```python
from build123d import *

# Parameters (mm, degrees)
CONG_1_R = 0.3


with BuildPart() as part:
    # Esquisse1 → Base-Révolution (revolve)
    with BuildSketch(Plane.XY):
        with BuildLine():
            Line((3.618033989, 3.25), (5, 3.25))
            Line((5, 3.25), (5, 2))
            Line((5, 2), (0, 2))
            Line((0, 2), (0, 3.25))
            Line((0, 3.25), (1.381966011, 3.25))
            ThreePointArc((1.381966011, 3.25), (2.5, 2.75), (3.618033989, 3.25))
        make_face()
    revolve(axis=Axis((0, 0, 0), (1, 0, 0)))

    # Congé1
    cong_1_edges = [part.edges().sort_by_distance(p)[0] for p in [
        (5, -2, 0),
        (0, -2, 0),
    ]]
    fillet(cong_1_edges, radius=CONG_1_R)


solid = part.part
```
Could you check a few things on this model? Use its own coordinates, in mm. Coordinates: 2 decimals unless noted, no trailing zeros. Write each loop counter-clockwise with the first axis right and the second up, starting at its lowest first coordinate (ties: lowest second). Pieces come first, ordered by that corner, then holes. Notation, with made-up numbers: (79.25, 28) - (96.25, 28) arc R25 ccw to (96.25, 42) - close; hole circle Ø2 at (44.5, 81). An arc over 180 degrees is marked (long way). Use a Markdown table: item, result.
Q1. Imagine slicing it at A-A (z = 0). List the corners of the cut face in (x, y) for me, and give its area (3 significant figures).
Geometry check:
| item | result |
|---|---|
| outline | (0, -3.25) - (1.38, -3.25) arc R1.5 cw to (3.62, -3.25) - (5, -3.25) - (5, -2.3) arc R0.3 ccw to (4.7, -2) - (0.3, -2) arc R0.3 ccw to (0, -2.3) - close; (0, 2.3) arc R0.3 ccw to (0.3, 2) - (4.7, 2) arc R0.3 ccw to (5, 2.3) - (5, 3.25) - (3.62, 3.25) arc R1.5 cw to (1.38, 3.25) - (0, 3.25) - close |
| area | 10.9 mm2 |
Q2. Please list where these lines run through material, in increasing order: L1, parallel to Z at x = 1.6, y = -0.75; L2, parallel to Y at x = 2.35, z = 1.75; L3, parallel to Z at x = 3.5, y = -1.25.
Geometry check:
| item | result |
|---|---|
| L1 | z = -2.96 to -1.85, 1.85 to 2.96 |
| L2 | y = -2.13 to -0.97, 0.97 to 2.13 |
| L3 | z = -2.87 to -1.56, 1.56 to 2.87 |
Q3. Imagine slicing it at C-C (x = 1.05). List the corners of the cut face in (y, z) for me, and give its area (3 significant figures).
Geometry check:
| item | result |
|---|---|
| outline | circle Ø6.5 at (0, 0); hole circle Ø4 at (0, 0) |
| area | 20.6 mm2 |
Q4. Thinking about a two-plate mould opening in Y: for faces 1 (the cylindrical face through (2, 0, -2)), 2 (the flat face through (5, 1.4, -2.1)), 3 (the cylindrical face through (4.319, -2.579, -1.978)), which applies, +Y half, -Y half, draft (parallel to the pull), parting line (faces both ways), or undercut?
Geometry check:
| item | result |
|---|---|
| face 1 | undercut |
| face 2 | draft |
| face 3 | parting line |
Q5. Imagine slicing it at D-D (x = 1.6). List the corners of the cut face in (y, z) for me.
Geometry check:
| item | result |
|---|---|
| outline | circle Ø6.1 at (0, 0); hole circle Ø4 at (0, 0) |
